from build123d import *

# Parameters (mm, degrees)
SKETCH1_R           = 2.05
BOSS_EXTRUDE1_DEPTH = 3


with BuildPart() as part:
    # Sketch1 → Boss-Extrude1 (new body)
    with BuildSketch(Plane(origin=(0, 0, 0), x_dir=(1, 0, 0), z_dir=(0, 1, 0))):
        with BuildLine():
            Line((46, 20), (-46, 20))
            ThreePointArc((-46, 20), (-47.414213562, 19.414213562), (-48, 18))
            Line((-48, 18), (-48, 1))
            ThreePointArc((-48, 1), (-47.707106781, 0.292893219), (-47, 0))
            Line((-47, 0), (-17, 0))
            ThreePointArc((-17, 0), (-16.292893219, 0.292893219), (-16, 1))
            Line((-16, 1), (-16, 7))
            ThreePointArc((-16, 7), (-15.707106781, 7.707106781), (-15, 8))
            Line((-15, 8), (15, 8))
            ThreePointArc((15, 8), (15.707106781, 7.707106781), (16, 7))
            Line((16, 7), (16, 1))
            ThreePointArc((16, 1), (16.292893219, 0.292893219), (17, 0))
            Line((17, 0), (47, 0))
            ThreePointArc((47, 0), (47.707106781, 0.292893219), (48, 1))
            Line((48, 1), (48, 18))
            ThreePointArc((48, 18), (47.414213562, 19.414213562), (46, 20))
        make_face()
        with Locations(Location((32, 10.8, 0), (0, 0, 270))):
            Circle(SKETCH1_R, mode=Mode.SUBTRACT)
        with Locations(Location((-32, 10.8, 0), (0, 0, 90))):
            Circle(SKETCH1_R, mode=Mode.SUBTRACT)
    extrude(amount=BOSS_EXTRUDE1_DEPTH)


solid = part.part
Model file for the job. Use its own axes, mm. A direction names the side the tool comes from. Give positions to 0.01 mm unless a question says otherwise; leave off trailing zeros. Write each loop counter-clockwise with the first axis right and the second up, starting at its lowest first coordinate (ties: lowest second). Pieces come first, ordered by that corner, then holes. Notation, with made-up numbers: (15.25, 4) -> (26.25, 4) arc R27 cw to (26.25, 26) -> close; hole circle Ø8 at (83, 22.5). An arc over 180 degrees is marked (long way). Write item = value, one per line.
(1) Tool access for faces 5 (the face through (0, 1, -8)), 6 (the face through (47.43, 1.48, -19.4)): list every direction of +Z, -Z, +X, -X, +Y, -Y with a clear straight run to the whole face (end or side of a thin tool).
Determined:
face_5 = +Z, +Y, -Y
face_6 = -Z, +X, +Y, -Y
(2) Slice it at B-B, the plane z = -10.8. Give the cut face in (x, y), then the cut area to 3 significant figures.
Determined:
outline = (-48, 0) -> (-34.05, 0) -> (-34.05, 3) -> (-48, 3) -> close; (-29.95, 0) -> (29.95, 0) -> (29.95, 3) -> (-29.95, 3) -> close; (34.05, 0) -> (48, 0) -> (48, 3) -> (34.05, 3) -> close
area = 263 mm2
(3) Mould opens along Z. For faces 1 (the face through (1, 1, -20)), 2 (the face through (-1, 3, -10)), 3 (the face through (34.033, 1.479, -11.067)), 4 (the face through (-33.73, 1.48, -11.9)) say: released by +Z, released by -Z, zero draft, split by the parting line, or undercut.
Determined:
face_1 = released by -Z
face_2 = zero draft
face_3 = undercut
face_4 = undercut
(4) Slice it at C-C, the plane y = 2.45. Give the cut face in (x, z).
Determined:
outline = (-48, -18) arc R2 ccw to (-46, -20) -> (46, -20) arc R2 ccw to (48, -18) -> (48, -1) arc R1 ccw to (47, 0) -> (17, 0) arc R1 ccw to (16, -1) -> (16, -7) arc R1 cw to (15, -8) -> (-15, -8) arc R1 cw to (-16, -7) -> (-16, -1) arc R1 ccw to (-17, 0) -> (-47, 0) arc R1 ccw to (-48, -1) -> close; hole circle Ø4.1 at (-32, -10.8); hole circle Ø4.1 at (32, -10.8)
(5) Slice it at D-D, the plane x = 5. Give the cut face in (y, z).
Determined:
outline = (0, -20) -> (3, -20) -> (3, -8) -> (0, -8) -> close
(6) Slice it at A-A, the plane x = -32. Give the cut face in (y, z).
Determined:
outline = (0, -20) -> (3, -20) -> (3, -12.85) -> (0, -12.85) -> close; (0, -8.75) -> (3, -8.75) -> (3, 0) -> (0, 0) -> close
(7) Probe line 1 along X through (y, z) = (1.2, -10.8); line 2 along X through (y, z) = (1.55, -6.25); line 3 along X through (y, z) = (1.15, -10). List the from-to ranges inside material, lowest first.
Determined:
line_1 = -48 to -34.05, -29.95 to 29.95, 34.05 to 48
line_2 = -48 to -16, 16 to 48
line_3 = -48 to -33.89, -30.11 to 30.11, 33.89 to 48
